```python
from build123d import *

# Parameters (mm, degrees)
EXTRUDE_THIN1_DEPTH = 6


with BuildPart() as part:
    # Sketch1 → Extrude-Thin1 (new body)
    with BuildSketch(Plane(origin=(0, 0, 0), x_dir=(1, 0, 0), z_dir=(0, 1, 0))):
        with BuildLine():
            Line((531.62539661, -259.643481844), (363.12, -259.643481844))
            ThreePointArc((363.12, -259.643481844), (357.905794596, -261.80327644), (355.746, -267.017481844))
            Line((355.746, -267.017481844), (355.746, -294.767481844))
            ThreePointArc((355.746, -294.767481844), (350.38, -300.133481844), (345.014, -294.767481844))
            Line((345.014, -294.767481844), (345.014, -267.017481844))
            ThreePointArc((345.014, -267.017481844), (342.854205404, -261.80327644), (337.64, -259.643481844))
            Line((337.64, -259.643481844), (101.625, -259.643481844))
            Line((101.625, -259.643481844), (101.625, -261.023481844))
            Line((101.625, -261.023481844), (337.64, -261.023481844))
            ThreePointArc((337.64, -261.023481844), (341.878398046, -262.779083798), (343.634, -267.017481844))
            Line((343.634, -267.017481844), (343.634, -294.767481844))
            ThreePointArc((343.634, -294.767481844), (350.38, -301.513481844), (357.126, -294.767481844))
            Line((357.126, -294.767481844), (357.126, -267.017481844))
            ThreePointArc((357.126, -267.017481844), (358.881601954, -262.779083798), (363.12, -261.023481844))
            Line((363.12, -261.023481844), (531.62539661, -261.023481844))
            Line((531.62539661, -261.023481844), (531.62539661, -259.643481844))
        make_face()
    extrude(amount=EXTRUDE_THIN1_DEPTH)


solid = part.part
```
Build history of the part. All positions in model axes, mm. A direction names the side the tool comes from. Coordinates: 2 decimals unless noted, no trailing zeros. Order: outer loops, then holes, each group sorted by start corner. A loop starts at its lowest first (then second) coordinate and runs counter-clockwise, first axis right, second up. Notation, with made-up numbers: M 0.25,-7.5 L 53.25,-7.5 A16 cw 53.25,4.5 Z; hole C 69.25,48 d8. An arc over 180 degrees is marked long. One line per question, with ' | ' between items. Start each with the question number.
1. Cut at C-C (x = 350.38). Write the cut outline in (y, z).
2. Cut at B-B (y = 4). Write the cut outline in (x, z) (3 decimals).
3. Tool access for faces 1 (the face through (316, 0, 260)), 2 (the face through (357.96, 2.96, 261.75)): list every direction of +Z, -Z, +X, -X, +Y, -Y with a clear straight run to the whole face (end or side of a thin tool).
4. Cut at A-A (z = 275.5). Write the cut outline in (x, y).
5. Flat gauge pins, fed straight in: P1, Ø3, axis at y = 3, z = 283.5, coming from the -X side; P2, Ø2, axis at x = 427.5, y = 3.5, coming from the +Z side; P3, Ø1.8, axis at y = 3, z = 287, coming from the +X side. Where does each tip first touch, or does it go through?
6. Mould opens along X. For faces 3 (the face through (342.91, 2.96, 261.86)), 4 (the face through (316, 6, 260)), 5 (the face through (350.23, 2.96, 301.51)) say: +X half, -X half, draft (parallel to the pull), parting line (faces both ways), or undercut.
7. Wall check: line 1 along X through (y, z) = (0.75, 271); line 2 along Z through (x, y) = (422, 5.75). Give the ranges that are in metal, low to high. Write a range as [from, to].
The answers:
1) outline: M 0,300.13 L 6,300.13 L 6,301.51 L 0,301.51 Z
2) outline: M 101.625,259.643 L 337.64,259.643 A7.374 ccw 345.014,267.017 L 345.014,294.767 A5.366 cw 355.746,294.767 L 355.746,267.017 A7.374 ccw 363.12,259.643 L 531.625,259.643 L 531.625,261.023 L 363.12,261.023 A5.994 cw 357.126,267.017 L 357.126,294.767 A6.746 ccw 343.634,294.767 L 343.634,267.017 A5.994 cw 337.64,261.023 L 101.625,261.023 Z
3) face 1: +Z, -Z, +X, -X, -Y | face 2: -Z, +Y, -Y
4) outline: M 343.63,0 L 345.01,0 L 345.01,6 L 343.63,6 Z; M 355.75,0 L 357.13,0 L 357.13,6 L 355.75,6 Z
5) P1: stops at x = 343.63 | P2: stops at z = 261.02 | P3: stops at x = 357.13
6) face 3: undercut | face 4: draft | face 5: parting line
7) line 1: x = [343.63, 345.01], [355.75, 357.13] | line 2: z = [259.64, 261.02]
